```python
from build123d import *

# Parameters (mm, degrees)
ESBO_O1_R                 = 4.9
RESSALTO_EXTRUS_O1_DEPTH  = 91
FURO_ROSCADO_DE_M51_D     = 4.2
FURO_ROSCADO_DE_M51_DEPTH = 12.7381927
FURO_ROSCADO_DE_M51_TIP   = 1.2618073
CORTE_EXTRUS_O1_DEPTH     = 8
CORTE_EXTRUS_O2_DEPTH     = 92.26346476
FURO_COM_FOLGA_DE_M21_D   = 2.4


with BuildPart() as part:
    # Esboço1 → Ressalto-extrusão1 (new body)
    with BuildSketch(Plane.XY):
        Circle(ESBO_O1_R)
    extrude(amount=RESSALTO_EXTRUS_O1_DEPTH)

    # Furo roscado de M51
    with Locations(Plane.XY.offset(91)):
        with Locations((0, 0)):
            Hole(FURO_ROSCADO_DE_M51_D / 2, depth=FURO_ROSCADO_DE_M51_DEPTH)
            with Locations((0, 0, -(FURO_ROSCADO_DE_M51_DEPTH + FURO_ROSCADO_DE_M51_TIP / 2))):  # 118° drill point
                Cone(0, FURO_ROSCADO_DE_M51_D / 2, FURO_ROSCADO_DE_M51_TIP, mode=Mode.SUBTRACT)

    # Esboço10 → Corte-extrusão1 (cut)
    with BuildSketch(Plane(origin=(0, 0, 0), x_dir=(-1, 0, 0), z_dir=(0, 0, -1))):
        with BuildLine():
            Line((-5, 0), (5, 0))
            ThreePointArc((5, 0), (0, 5), (-5, 0))
        make_face()
    extrude(amount=-CORTE_EXTRUS_O1_DEPTH, mode=Mode.SUBTRACT)

    # Esboço18 → Corte-extrusão2 (cut, through all)
    with BuildSketch(Plane(origin=(0, 0, 0), x_dir=(1, 0, 0), z_dir=(0, 1, 0))):
        with BuildLine():
            Line((-4.9, -2.002506281), (-4.9, 0))
            Line((-4.9, 0), (-2.45, 0))
            ThreePointArc((-2.45, 0), (-4.032129215, -0.564317395), (-4.9, -2.002506281))
        make_face()
        with BuildLine():
            Line((2.45, 0), (4.9, 0))
            Line((4.9, 0), (4.9, -2.002506281))
            ThreePointArc((4.9, -2.002506281), (4.032129215, -0.564317395), (2.45, 0))
        make_face()
    extrude(amount=-CORTE_EXTRUS_O2_DEPTH, mode=Mode.SUBTRACT)

    # Furo com folga de M21 (through all)
    with Locations(Plane(origin=(-3, 0, 3), x_dir=(0, 0, 1), z_dir=(0, 1, 0))):
        with Locations((0, 0), (0, 6)):
            Hole(FURO_COM_FOLGA_DE_M21_D / 2)


solid = part.part
```
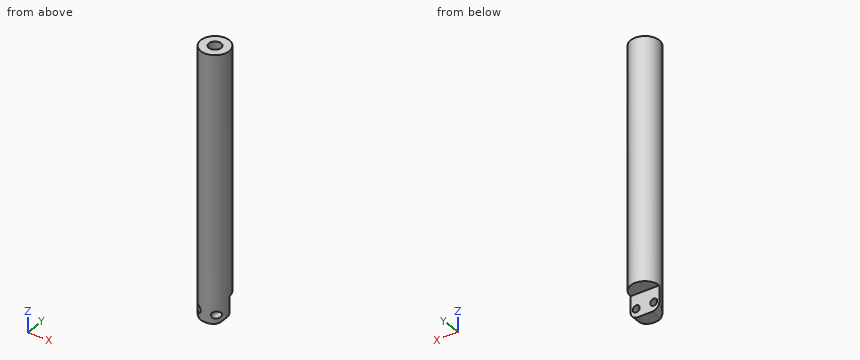
The model under review builds one solid part; all positions refer to its coordinate system, in mm. Round coordinates to 2 decimals unless told otherwise and drop trailing zeros. Loops run counter-clockwise (first coordinate to the right, second up) from the corner with the lowest first, then second, coordinate; pieces in that order, holes last.
1) Consider section C-C on y = 3.75. State the section outline as (x, z) points.
Values follow:
outline: (-3.15, 8) - (3.15, 8) - (3.15, 91) - (-3.15, 91) - close
2) Consider section A-A on z = 3. State the section outline as (x, y) points.
Values follow:
outline: (-4.9, 0) arc R4.9 ccw to (-4.2, -2.52) - (-4.2, 0) - close; (-1.8, -4.56) arc R4.9 ccw to (1.8, -4.56) - (1.8, 0) - (-1.8, 0) - close; (4.2, -2.52) arc R4.9 ccw to (4.9, 0) - (4.2, 0) - close
3) Wall thickness on line 1 along X through (y, z) = (-0.25, 85); line 2 along Y through (x, z) = (4.25, 40.5); line 3 along Z through (x, y) = (-0.25, 4.25): over which ranges is each line inside the solid? List them lowest first.
Values follow:
line 1: x = -4.89 to -2.09, 2.09 to 4.89
line 2: y = -2.44 to 2.44
line 3: z = 8 to 91
4) Clearance check with flat-ended pins moving along their axes: P1, Ø3, axis at x = 1.5, z = 12.5, coming from the -Y side; P2, Ø1.5, axis at x = -1, y = 3, coming from the -Z side; P3, Ø2, axis at x = -3, z = 3, coming from the +Y side; P4, Ø3, axis at x = 3, z = 3, coming from the -Y side. State where each tip first meets the part, or that it passes through.
Values follow:
P1: stops at y = -4.9
P2: stops at z = 8
P3: passes through
P4: stops at y = -4.66
5) Consider section B-B on z = 48.5. State the section outline as (x, y) points, then the cut area to 3 significant figures.
Values follow:
outline: circle Ø9.8 at (0, 0)
area: 75.4 mm2
